```python
from build123d import *

# Parameters (mm, degrees)
BOSS_EXTRUDE1_DEPTH = 2
FILLET1_R           = 0.25
SKETCH3_W           = 26
SKETCH3_H           = 12
CUT_EXTRUDE2_DEPTH  = 1
FILLET6_R           = 2
SKETCH4_W           = 36.903708965
SKETCH4_H           = 12
CUT_EXTRUDE3_DEPTH  = 5
BOSS_EXTRUDE2_DEPTH = 6


with BuildPart() as part:
    # Sketch1 → Boss-Extrude1 (new body)
    with BuildSketch(Plane(origin=(0, 0, 0), x_dir=(1, 0, 0), z_dir=(0, 1, 0))):
        Polygon((-15, 2.618365096), (-20, 3.5), (-20, -3.5), (-15, -2.618365096), (-15, -6), (15, -6), (15, -2.618365096), (20, -3.5), (20, 3.5), (15, 2.618365096), (15, 6), (-15, 6), align=None)
    extrude(amount=BOSS_EXTRUDE1_DEPTH)

    # Fillet1
    fillet1_edges = [part.edges().sort_by_distance(p)[0] for p in [
        (15, 1, -2.618365096),
        (20, 1, -3.5),
        (20, 1, 3.5),
        (15, 1, 2.618365096),
        (-15, 1, 2.618365096),
        (-20, 1, 3.5),
        (-20, 1, -3.5),
        (-15, 1, -2.618365096),
    ]]
    fillet(fillet1_edges, radius=FILLET1_R)

    # Sketch3 → Cut-Extrude2 (cut)
    with BuildSketch(Plane(origin=(0, 2, 0), x_dir=(1, 0, 0), z_dir=(0, 1, 0))):
        Rectangle(SKETCH3_W, SKETCH3_H)
    extrude(amount=-CUT_EXTRUDE2_DEPTH, mode=Mode.SUBTRACT)

    # Fillet6
    # the kernel refuses this fillet: 2 mm, written as the material it adds along each edge
    with BuildSketch(Plane(origin=(-13, 1, 6), x_dir=(0, 1, 0), z_dir=(0, 0, -1))) as fillet6_piece_1:
        with BuildLine():
            CenterArc((2, 1.732050808), FILLET6_R, 180, 60)
            Line((0, 1.732050808), (-0.04, 1.732050808))
            Line((-0.04, 1.732050808), (-0.04, 0))
            Line((-0.04, 0), (0, -0.04))
            ThreePointArc((0, -0.04), (0.5, -0.04), (0.98, -0.034641016))
            Line((0.98, -0.034641016), (1, 0))
        make_face()
    extrude(amount=12)
    with BuildSketch(Plane(origin=(13, 1, -6), x_dir=(-1, 0, 0), z_dir=(0, 0, 1))) as fillet6_piece_2:
        with BuildLine():
            CenterArc((1.732050808, -2), FILLET6_R, 90, 60)
            Line((0, -1), (-0.034641016, -0.98))
            ThreePointArc((-0.034641016, -0.98), (-0.04, -0.5), (-0.04, 0))
            Line((-0.04, 0), (0, 0.04))
            Line((0, 0.04), (1.732050808, 0.04))
            Line((1.732050808, 0.04), (1.732050808, 0))
        make_face()
    extrude(amount=12)

    # Sketch4 → Cut-Extrude3 (cut, symmetric)
    with BuildSketch(Plane(origin=(0, 1, 0), x_dir=(1, 0, 0), z_dir=(0, 1, 0))):
        with Locations((7.18390529, 0)):
            Rectangle(SKETCH4_W, SKETCH4_H)
    extrude(amount=CUT_EXTRUDE3_DEPTH, both=True, mode=Mode.SUBTRACT)

    # Sketch6 → Boss-Extrude2 (add, symmetric)
    with BuildSketch(Plane.XY):
        with BuildLine():
            Line((-11.267949192, 0), (-11.267949192, 1))
            Line((-11.267949192, 1), (-6.267949192, 1))
            ThreePointArc((-6.267949192, 1), (-2.202085201, 2.684136008), (-0.517949192, 6.75))
            Line((-0.517949192, 6.75), (0.482050808, 6.75))
            ThreePointArc((0.482050808, 6.75), (-1.494978419, 1.977029227), (-6.267949192, 0))
            Line((-6.267949192, 0), (-11.267949192, 0))
        make_face()
    extrude(amount=BOSS_EXTRUDE2_DEPTH, both=True)

    # Mirror3: part across plane


with BuildPart() as part_1:
    add(part.part)
    add(part.part.mirror(Plane.ZX.offset(6.75)))


solid = part_1.part
```
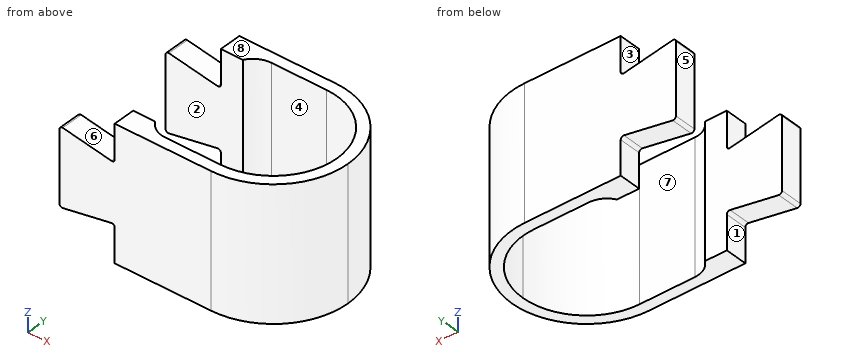
CAD build for the part. Positions are in the model's coordinates, mm. Face numbers are marked on the shaded views. A direction names the side the tool comes from. Round coordinates to 2 decimals unless told otherwise and drop trailing zeros. Order: outer loops, then holes, each group sorted by start corner. A loop starts at its lowest first (then second) coordinate and runs counter-clockwise, first axis right, second up. Notation, with made-up numbers: (71, 13.5) - (127, 13.5) arc R6 ccw to (127, 17.5) - close; hole circle Ø11 at (15, 65.25). An arc over 180 degrees is marked (long way). Answer in a Markdown table with one row per item. Add a question column.
(1) 3-axis set-ups, long thin cutter, end or side, ignore diameter. For the marked faces 1, 2, 3 and 4: which of +Z, -Z, +X, -X, +Y, -Y reach the whole face in a straight line?
(2) Drop flat-ended pins along their axis: pin 1 Ø1 at (y, z) = (1.5, -4.5) entering from -X; pin 2 Ø1.5 at (y, z) = (8.5, 3) entering from +X. Give the stop position or say it passes through.
(3) Band-saw the part on D-D on y = 7.75. List the corners of the cut face in (x, z).
(4) Band-saw the part on C-C on z = 1.75. List the corners of the cut face in (x, y).
(5) Band-saw the part on A-A on x = -14.75. List the corners of the cut face in (y, z), and give its area (3 significant figures).
(6) Probe L1, parallel to Y at x = -15.25, z = 2; L2, parallel to Y at x = -7.25, z = -4; L3, parallel to X at y = 6.5, z = -3.25. List the from-to ranges inside material, lowest first. Write a range as [from, to].
(7) Mould opens along X. For the marked faces 5, 6, 7 and 8 say: +X half, -X half, draft (parallel to the pull), parting line (faces both ways), or undercut.
(8) Band-saw the part on B-B on x = -9.25. List the corners of the cut face in (y, z), and give its area (3 significant figures).
Data:
| question | item | result |
|---|---|---|
| 1 | face 1 | -Z, +Y, -Y |
| 1 | face 2 | +Z, -Z, -X |
| 1 | face 3 | +Z, +Y, -Y |
| 1 | face 4 | +Z, -Z |
| 2 | pin 1 | stops at x = -15 |
| 2 | pin 2 | stops at x = 0.41 |
| 3 | outline | (-0.61, -6) - (0.41, -6) - (0.41, 6) - (-0.61, 6) - close |
| 4 | outline | (-20, 0) - (-6.27, 0) arc R6.75 ccw to (-6.27, 13.5) - (-20, 13.5) - (-20, 11.5) - (-13, 11.5) arc R2 cw to (-11.27, 12.5) - (-6.27, 12.5) arc R5.75 cw to (-6.27, 1) - (-11.27, 1) arc R2 cw to (-13, 2) - (-20, 2) - close |
| 5 | outline | (0, -6) - (2, -6) - (2, 6) - (0, 6) - close; (11.5, -6) - (13.5, -6) - (13.5, 6) - (11.5, 6) - close |
| 5 | area | 48.0 mm^2 |
| 6 | L1 | y = [0, 2], [11.5, 13.5] |
| 6 | L2 | y = [0, 1], [12.5, 13.5] |
| 6 | L3 | x = [-0.52, 0.48] |
| 7 | face 5 | -X half |
| 7 | face 6 | undercut |
| 7 | face 7 | undercut |
| 7 | face 8 | draft |
| 8 | outline | (0, -6) - (1, -6) - (1, 6) - (0, 6) - close; (12.5, -6) - (13.5, -6) - (13.5, 6) - (12.5, 6) - close |
| 8 | area | 24.0 mm^2 |
